Verification items for the finished model (mm, model axes). Face numbers are marked on the shaded views. Round coordinates to 2 decimals unless told otherwise and drop trailing zeros. Order: outer loops, then holes, each group sorted by start corner. A loop starts at its lowest first (then second) coordinate and runs counter-clockwise, first axis right, second up. Notation, with made-up numbers: M 58.5,79 L 76.5,79 A9 cw 76.5,95 Z; hole C 32,59.25 d3. An arc over 180 degrees is marked long. Use one line per item in the form item = value. Start each with the question number.
Item 1: Release check for a two-part mould opening along Z. For the marked faces 1, 2 and 3 record: +Z half, -Z half, draft (parallel to the pull), parting line (faces both ways), or undercut.
Item 2: Cross-section at A-A on y = -1.9. Enter the section's corners in (x, z), then the cut area to 3 significant figures.
Item 3: Go/stop test with flat-tipped pins: pin 1 Ø2 at (x, z) = (0, 0.5) entering from +Y; pin 2 Ø3.5 at (y, z) = (0, 0) entering from -X. Record where each tip stops, or that it passes through.
Item 4: Cross-section at B-B on x = -1.25. Enter the section's corners in (y, z), then the cut area to 3 significant figures.
Item 5: Thickness scan on probe 1 along Y at (x, z) = (-1.25, 0); probe 2 along Z at (x, y) = (-0.75, 1.4); probe 3 along Y at (x, z) = (0, 2). Record the ranges inside material, lowest first. Write a range as [from, to].
Item 6: Cross-section at C-C on z = 1.8. Count the separate pieces of the cut face and the enclosed holes in it, then the cut area to 3 significant figures.
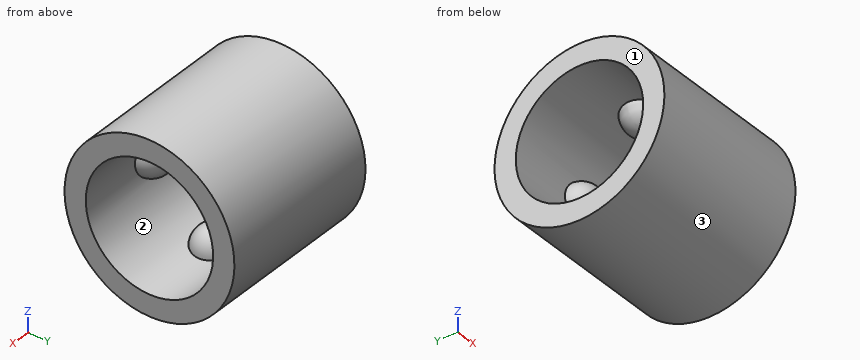
from build123d import *

# Parameters (mm, degrees)
SKETCH2_R           = 3
SKETCH2_R_2         = 2.25
BOSS_EXTRUDE1_DEPTH = 3


with BuildPart() as part:
    # Sketch2 → Boss-Extrude1 (new, symmetric)
    with BuildSketch(Plane(origin=(0, 0, 0), x_dir=(0, 0, -1), z_dir=(1, 0, 0))):
        Circle(SKETCH2_R)
        Circle(SKETCH2_R_2, mode=Mode.SUBTRACT)
    extrude(amount=BOSS_EXTRUDE1_DEPTH, both=True)

    # Sketch8 → Revolve18 (revolve)
    with BuildSketch(Plane(origin=(0, 0, 0), x_dir=(0, 0, -1), z_dir=(1, 0, 0))):
        with BuildLine():
            Line((-2.25, 0), (-2.237739596, 0.750859778))
            ThreePointArc((-2.237739596, 0.750859778), (-1.7107227, 0.52222122), (-1.500084905, -0.012244979))
            Line((-1.500084905, -0.012244979), (-2.25, 0))
        make_face()
    revolve(axis=Axis((0, 0, 2.25), (0, -0.016326311142728266, -0.999866716900043)))

    # Sketch10 → Revolve19 (revolve)
    with BuildSketch(Plane(origin=(0, 0, 0), x_dir=(0, 0, -1), z_dir=(1, 0, 0))):
        with BuildLine():
            Line((2.25, 0), (2.25, 0.75))
            ThreePointArc((2.25, 0.75), (1.719669914, 0.530330086), (1.5, 0))
            Line((1.5, 0), (2.25, 0))
        make_face()
    revolve(axis=Axis((0, 0, -2.25), (0, 0, 1)))


with BuildPart() as revolve20_tool:
    # Sketch11 → Revolve20 (revolve)
    with BuildSketch(Plane(origin=(0, 0, 0), x_dir=(0, 0, -1), z_dir=(1, 0, 0))):
        with BuildLine():
            Line((0.001073711, 2.249994313), (-0.749995081, 2.251069562))
            ThreePointArc((-0.749995081, 2.251069562), (-0.53070663, 1.720048449), (0, 1.5))
            Line((0, 1.5), (0.001073711, 2.249994313))
        make_face()
    revolve(axis=Axis((0, 2.249994313, -0.001073711), (0, -0.9999989752258402, 0.0014316239972306517)))


with BuildPart() as part_1:
    add(part.part)


with BuildPart() as part_2:
    # Revolve20: joined with revolve20_tool
    add(part_1.part.fuse(revolve20_tool.part, tol=0.00001))

    # Sketch13 → Revolve21 (revolve)
    with BuildSketch(Plane(origin=(0, 0, 0), x_dir=(0, 0, -1), z_dir=(1, 0, 0))):
        with BuildLine():
            Line((0, -1.5), (0, -2.25))
            Line((0, -2.25), (0.75, -2.25))
            ThreePointArc((0.75, -2.25), (0.530330086, -1.719669914), (0, -1.5))
        make_face()
    revolve(axis=Axis((0, -1.5, 0), (0, -1, 0)))


solid = part_2.part
Output values:
q1.face_1 = draft
q1.face_2 = undercut
q1.face_3 = parting line
q2.outline = M -3,-2.32 L 3,-2.32 L 3,-1.21 L -3,-1.21 Z; M -3,1.21 L 3,1.21 L 3,2.32 L -3,2.32 Z; C 0,0 d1.33
q2.area = 14.8 mm2
q3.pin_1 = 3
q3.pin_2 = -0.56
q4.outline = C 0,0 d6; hole C 0,0 d4.5
q4.area = 12.4 mm2
q5.probe_1 = [-3, -2.25], [2.25, 3]
q5.probe_2 = [-2.65, -1.76], [1.76, 2.65]
q5.probe_3 = [-2.24, -1.03], [-0.71, 0.71], [1.03, 2.24]
q6.separate_pieces = 3
q6.enclosed_holes = 0
q6.area = 13.7 mm2
